Check sheet for the drawn part. Datum: minimum x, y, z corner. Units: mm. A direction names the side the tool comes from. Give positions to 0.01 mm unless a question says otherwise; leave off trailing zeros. Write each loop counter-clockwise with the first axis right and the second up, starting at its lowest first coordinate (ties: lowest second). Pieces come first, ordered by that corner, then holes.
(1) Tool access check on the marked faces 1 and 2. Record the directions out of +Z, -Z, +X, -X, +Y, -Y that give a thin tool (end or side, any length) a straight path to the whole face; none if there is none.
(2) Cross-section at C-C (z = 2.75). Record the boundary of the cut face in (x, y), and give its area (3 significant figures).
(3) Depth check by flat-ended pin: P1, Ø1.5, axis at x = 7, y = 2, coming from the +Z side. Enter the tip coordinate at first touch or a pass-through.
(4) Cross-section at D-D (z = 0.75). Record the boundary of the cut face in (x, y).
(5) Thickness scan on line 1 along Z through (x, y) = (10.25, 6.5); line 2 along Y through (x, z) = (6, 4.5); line 3 along X through (y, z) = (9, 0.2). Record the ranges inside material, lowest first.
(6) Cross-section at A-A (y = 6). Record the boundary of the cut face in (x, z), and give its area (3 significant figures).
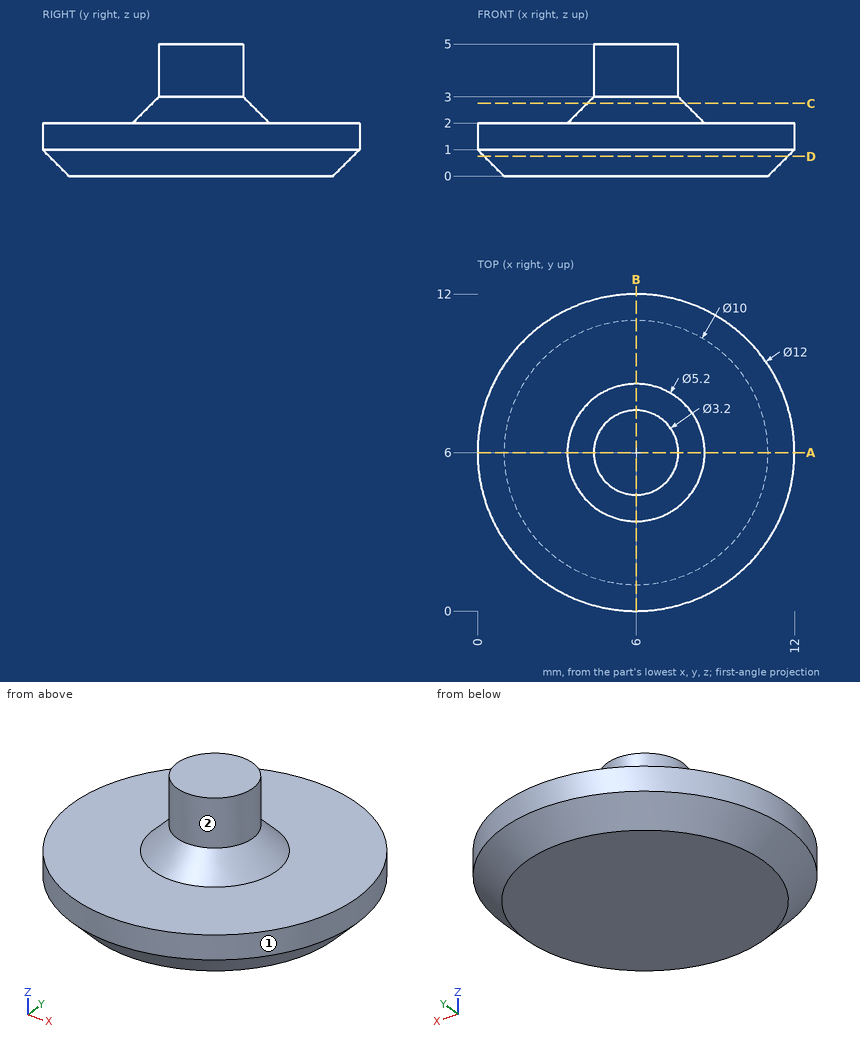
Reply:
1. face 1: +Z, -Z
1. face 2: +Z
2. outline: circle Ø3.7 at (6, 6)
2. area: 10.8 mm2
3. P1: stops at z = 2
4. outline: circle Ø11.5 at (6, 6)
5. line 1: z = 0 to 2
5. line 2: y = 4.4 to 7.6
5. line 3: x = 1.75 to 10.25
6. outline: (0, 1) - (1, 0) - (11, 0) - (12, 1) - (12, 2) - (8.6, 2) - (7.6, 3) - (7.6, 5) - (4.4, 5) - (4.4, 3) - (3.4, 2) - (0, 2) - close
6. area: 33.6 mm2
